Geometry: final body of the model. Coordinates: model frame, mm. Face numbers are marked on the shaded views. A direction names the side the tool comes from. Round coordinates to 2 decimals unless told otherwise and drop trailing zeros. Order: outer loops, then holes, each group sorted by start corner. A loop starts at its lowest first (then second) coordinate and runs counter-clockwise, first axis right, second up. Notation, with made-up numbers: M 52,85.5 L 89,85.5 A32 ccw 89,114.5 Z; hole C 79.5,73 d10. An arc over 180 degrees is marked long. Put each result on its own line as item: value. Start each with the question number.
1) Material intervals for probe 1 along Y at (x, z) = (0, 4.8); probe 2 along Y at (x, z) = (13.5, 1.95); probe 3 along X at (y, z) = (-12, 1.6), sorted ascending. Write a range as [from, to].
2) Section D-D, the plane x = -31. Return loops of the section in (y, z).
3) Access query for the marked faces 4 and 5. Directions: +Z, -Z, +X, -X, +Y, -Y. A direction counts if a zero-diameter tool reaches every point of the face in a straight line with its end or side. Return the directions, or none.
4) Draft query along X for the marked faces 1, 2 and 3. Return one class per face: pulls with the +X half, pulls with the -X half, needs draft (parallel to the pull), parting line crosses it, or undercut.
5) Section C-C, the plane z = 5. Return loops of the section in (x, y), then the cut area to 3 significant figures.
6) Section A-A, the plane x = 0. Return loops of the section in (y, z).
7) First-contact query: P1, Ø1.5, axis at y = 4.5, z = 4, coming from the -X side; P2, Ø1.5, axis at x = 18.5, y = 30, coming from the +Z side; P3, Ø1.5, axis at y = -25.5, z = 5, coming from the +X side. Flat tips, straight axial feed; report the tip coordinate or a pass-through.
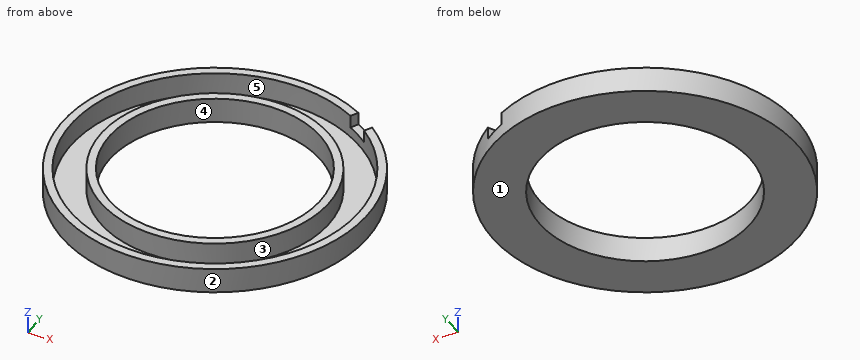
from build123d import *

# Parameters (mm, degrees)
SKETCH1_R             = 36
SKETCH1_R_2           = 34
BOSS_EXTRUDE1_DEPTH   = 6
SKETCH1_R_3           = 26.9
SKETCH1_R_4           = 24.9
BOSS_EXTRUDE1_2_DEPTH = 6
SKETCH1_3_R           = 34
SKETCH1_3_R_2         = 26.9
BOSS_EXTRUDE2_DEPTH   = 0.6
CUT_EXTRUDE1_DEPTH    = 3


with BuildPart() as part:
    # Sketch1 → Boss-Extrude1 (new body)
    with BuildSketch(Plane.XY):
        Circle(SKETCH1_R)
        Circle(SKETCH1_R_2, mode=Mode.SUBTRACT)
    extrude(amount=BOSS_EXTRUDE1_DEPTH)



with BuildPart() as body_2:
    # Sketch1 → Boss-Extrude1 2 (new body)
    with BuildSketch(Plane.XY):
        Circle(SKETCH1_R_3)
        Circle(SKETCH1_R_4, mode=Mode.SUBTRACT)
    extrude(amount=BOSS_EXTRUDE1_2_DEPTH)


with BuildPart() as part_1:
    add(part.part)

    add(body_2.part)  # Boss-Extrude2 merges body 2
    # Sketch1<3> → Boss-Extrude2 (add)
    with BuildSketch(Plane.XY):
        Circle(SKETCH1_3_R)
        Circle(SKETCH1_3_R_2, mode=Mode.SUBTRACT)
    extrude(amount=BOSS_EXTRUDE2_DEPTH)

    # Sketch4 → Cut-Extrude1 (cut)
    with BuildSketch(Plane.XY.offset(6)):
        Polygon((22.015125438, 28.483929714), (21.055768183, 26.695591888), (17.287744391, 26.985727401), (16.035297847, 29.981147793), (16.978550661, 31.744744722), (21.055768183, 32.257714182), align=None)
    extrude(amount=-CUT_EXTRUDE1_DEPTH, mode=Mode.SUBTRACT)


solid = part_1.part
Result sheet:
1. probe 1: y = [-36, -34], [-26.9, -24.9], [24.9, 26.9], [34, 36]
1. probe 2: y = [-33.37, -31.2], [-23.27, -20.92], [20.92, 23.27], [31.2, 33.37]
1. probe 3: x = [-33.94, -31.81], [-24.08, -21.82], [21.82, 24.08], [31.81, 33.94]
2. outline: M -18.3,0 L 18.3,0 L 18.3,6 L 13.96,6 L 13.96,0.6 L -13.96,0.6 L -13.96,6 L -18.3,6 Z
3. face 4: +Z, -Z
3. face 5: +Z
4. face 1: needs draft
4. face 2: parting line crosses it
4. face 3: undercut
5. outline: C 0,0 d53.8; M 16.04,29.98 L 16.98,31.74 A36 ccw long 22.02,28.48 L 21.06,26.7 A34 cw long Z; hole C 0,0 d49.8
5. area: 753 mm2
6. outline: M -36,0 L -24.9,0 L -24.9,6 L -26.9,6 L -26.9,0.6 L -34,0.6 L -34,6 L -36,6 Z; M 24.9,0 L 36,0 L 36,6 L 34,6 L 34,0.6 L 26.9,0.6 L 26.9,6 L 24.9,6 Z
7. P1: stops at x = -35.8
7. P2: stops at z = 3
7. P3: stops at x = 26.14
